from build123d import *

# Parameters (mm, degrees)
SKETCH_1_R          = 10
SKETCH_1_R_2        = 4
EXTRUDE_1_DEPTH     = 20
SKETCH_2_W          = 1
SKETCH_2_H          = 20
CUT_EXTRUDE_1_DEPTH = 25.494897428


with BuildPart() as part:
    # ｽｹｯﾁ1 → ﾎﾞｽ - 押し出し1 (new body)
    with BuildSketch(Plane(origin=(0, 0, 0), x_dir=(0, 0, -1), z_dir=(1, 0, 0))):
        Circle(SKETCH_1_R)
        Circle(SKETCH_1_R_2, mode=Mode.SUBTRACT)
    extrude(amount=EXTRUDE_1_DEPTH)

    # ｽｹｯﾁ2 → ｶｯﾄ - 押し出し1 (cut, through all)
    with BuildSketch(Plane(origin=(0, 0, 0), x_dir=(1, 0, 0), z_dir=(0, 1, 0))):
        with Locations((10, 0)):
            Rectangle(SKETCH_2_W, SKETCH_2_H)
    extrude(amount=CUT_EXTRUDE_1_DEPTH, mode=Mode.SUBTRACT)


solid = part.part
The model under review builds one solid part; all positions refer to its coordinate system, in mm. A direction names the side the tool comes from. Coordinates: 2 decimals unless noted, no trailing zeros. Order: outer loops, then holes, each group sorted by start corner. A loop starts at its lowest first (then second) coordinate and runs counter-clockwise, first axis right, second up. Notation, with made-up numbers: (-37.5, -28.5) -> (0.5, -28.5) arc R26 cw to (0.5, 4.5) -> close; hole circle Ø9 at (-5, 61). An arc over 180 degrees is marked (long way). Answer in a Markdown table with one row per item.
(1) Consider section A-A (y = 6). Write out the cut boundary in (x, z).
Answers:
| item | result |
|---|---|
| outline | (0, -8) -> (9.5, -8) -> (9.5, 8) -> (0, 8) -> close; (10.5, -8) -> (20, -8) -> (20, 8) -> (10.5, 8) -> close |
(2) Wall thickness on line 1 along Z through (x, y) = (7, 0); line 2 along X through (y, z) = (4.75, -7.5): over which ranges is each line inside the solid? List them lowest first.
Answers:
| item | result |
|---|---|
| line 1 | -10 to -4, 4 to 10 |
| line 2 | 0 to 9.5, 10.5 to 20 |
(3) The part is to be moulded in two halves that separate along Z. For faces 3 (the flat face through (20, -4.3, 0.1)), 4 (the cylindrical face through (9.86, -3.905, 0.867)), 5 (the cylindrical face through (9.86, -9.76, 2.17)), say which applies: +Z half, -Z half, draft (parallel to the pull), parting line (faces both ways), or undercut.
Answers:
| item | result |
|---|---|
| face 3 | draft |
| face 4 | undercut |
| face 5 | parting line |
(4) Consider section B-B (z = 0). Write out the cut boundary in (x, y), plus the area to 3 significant figures.
Answers:
| item | result |
|---|---|
| outline | (0, -10) -> (20, -10) -> (20, -4) -> (0, -4) -> close; (0, 4) -> (9.5, 4) -> (9.5, 10) -> (0, 10) -> close; (10.5, 4) -> (20, 4) -> (20, 10) -> (10.5, 10) -> close |
| area | 234 mm² |
(5) Consider section D-D (x = 16.5). Write out the cut boundary in (y, z).
Answers:
| item | result |
|---|---|
| outline | circle Ø20 at (0, 0); hole circle Ø8 at (0, 0) |
(6) Consider section C-C (y = 1.75). Write out the cut boundary in (x, z), plus the area to 3 significant figures.
Answers:
| item | result |
|---|---|
| outline | (0, -9.85) -> (9.5, -9.85) -> (9.5, -3.6) -> (0, -3.6) -> close; (0, 3.6) -> (9.5, 3.6) -> (9.5, 9.85) -> (0, 9.85) -> close; (10.5, -9.85) -> (20, -9.85) -> (20, -3.6) -> (10.5, -3.6) -> close; (10.5, 3.6) -> (20, 3.6) -> (20, 9.85) -> (10.5, 9.85) -> close |
| area | 237 mm² |
(7) Machinability: for faces 1 (the flat face through (0, -4.3, 0.1)), 2 (the flat face through (10, 0, -7)), which of the approach directions +Z, -Z, +X, -X, +Y, -Y give a long, thin tool a straight path to every point of the face, cutting with its end or side? Answer none if there is none.
Answers:
| item | result |
|---|---|
| face 1 | +Z, -Z, -X, +Y, -Y |
| face 2 | +Z, -Z, +Y |
(8) Insertion check: pin 1 (1.5 mm diameter, centred on x = 14, y = -2, fed in from -Z); pin 2 (0.8 mm diameter, centred on x = 10, z = 6.5, fed in from +Y). Each pin has a flat end and moves straight along its axis. Give the tip position at first contact, or say it passes through.
Answers:
| item | result |
|---|---|
| pin 1 | z = -9.92 |
| pin 2 | y = 0 |
